Model file for the job. Use its own axes, mm. A direction names the side the tool comes from. Round coordinates to 2 decimals unless told otherwise and drop trailing zeros. Loops run counter-clockwise (first coordinate to the right, second up) from the corner with the lowest first, then second, coordinate; pieces in that order, holes last. Notation, with made-up numbers: M 78,54 L 114,54 A13 ccw 114,64 Z; hole C -15.5,50.25 d3. An arc over 180 degrees is marked long. Use a Markdown table: item, result. Add a question column.
Q1. Cut at D-D (x = 22). Give the cut face in (y, z).
Q2. Pin check, flat tips, straight feed: pin 1 (2 mm diameter, centred on x = 55, z = 23, fed in from -Y); pin 2 (20.5 mm diameter, centred on y = 32.5, z = 25, fed in from +X); pin 3 (1.5 mm diameter, centred on y = 52, z = 41, fed in from +X); pin 4 (8.5 mm diameter, centred on x = 49.6, z = 37.7, fed in from +Y). Stop position of each tip, or through.
Q3. Cut at A-A (z = 25). Give the cut face in (x, y) (3 decimals), plus the area to 3 significant figures.
Q4. Tool access for faces 4 (the face through (40, 2.997, 25)), 5 (the face through (41, 0, 25)): list every direction of +Z, -Z, +X, -X, +Y, -Y with a clear straight run to the whole face (end or side of a thin tool).
Q5. Probe line 1 (X direction, y = 42, z = 13.5); line 2 (Y direction, x = 1.65, z = 46.19). List the from-to ranges inside material, lowest first. Write a range as from..to.
Q6. Cut at B-B (y = 23.5). Give the cut face in (x, z), plus the area to 3 significant figures.
Q7. Cut at C-C (z = 30). Give the cut face in (x, y) (3 decimals), plus the area to 3 significant figures.
Q8. Mould opens along Y. For faces 1 (the face through (1, 59.995, 25)), 2 (the face through (21, 1, 50)), 3 (the face through (1.478, 21.233, 30.86)) say: +Y half, -Y half, draft (parallel to the pull), parting line (faces both ways), or undercut.
from build123d import *

# Parameters (mm, degrees)
BOSS_EXTRUDE1_DEPTH       = 50
SKETCH5_R                 = 3.2639
MOUNTING_HORIZONTAL_DEPTH = 107.647674169
SKETCH7_R                 = 12.7
BEARING_WITH_MOTOR_DEPTH  = 109.279157861
SKETCH8_R                 = 1.4732
F_4_40_WITH_MOTOR_DEPTH   = 109.279157861


with BuildPart() as part:
    # Sketch2 → Boss-Extrude1 (new body)
    with BuildSketch(Plane.XY):
        with BuildLine():
            Line((0, 5.842), (0, 59.9948))
            Line((0, 59.9948), (2.9972, 59.9948))
            Line((2.9972, 59.9948), (2.9972, 6.1722))
            ThreePointArc((2.9972, 6.1722), (3.92713597, 3.92713597), (6.1722, 2.9972))
            Line((6.1722, 2.9972), (75, 2.9972))
            Line((75, 2.9972), (75, 0))
            Line((75, 0), (5.842, 0))
            ThreePointArc((5.842, 0), (1.711082184, 1.711082184), (0, 5.842))
        make_face()
    extrude(amount=BOSS_EXTRUDE1_DEPTH)

    # Sketch5 → Mounting -- Horizontal (cut, through all)
    with BuildSketch(Plane(origin=(0, 2.9972, 0), x_dir=(1, 0, 0), z_dir=(0, 1, 0))):
        with Locations(Location((49.6, -12.3, 0), (0, 0, 270))):
            Circle(SKETCH5_R)
        with Locations(Location((49.6, -37.7, 0), (0, 0, 270))):
            Circle(SKETCH5_R)
    extrude(amount=-MOUNTING_HORIZONTAL_DEPTH, mode=Mode.SUBTRACT)

    # Sketch7 → Bearing -- With Motor (cut, through all)
    with BuildSketch(Plane.ZY):
        with Locations((25, 32.5)):
            Circle(SKETCH7_R)
    extrude(amount=-BEARING_WITH_MOTOR_DEPTH, mode=Mode.SUBTRACT)

    # Sketch8 → 4-40 -- With Motor (cut, through all)
    with BuildSketch(Plane.ZY):
        with Locations((3.81, 32.5)):
            Circle(SKETCH8_R)
        with Locations((46.19, 32.5)):
            Circle(SKETCH8_R)
    extrude(amount=-F_4_40_WITH_MOTOR_DEPTH, mode=Mode.SUBTRACT)


solid = part.part
Checked values:
| question | item | result |
|---|---|---|
| 1 | outline | M 0,0 L 3,0 L 3,50 L 0,50 Z |
| 2 | pin 1 | stops at y = 0 |
| 2 | pin 2 | passes through |
| 2 | pin 3 | stops at x = 3 |
| 2 | pin 4 | stops at y = 3 |
| 3 | outline | M 0,5.842 A5.842 ccw 5.842,0 L 75,0 L 75,2.997 L 6.172,2.997 A3.175 cw 2.997,6.172 L 2.997,19.8 L 0,19.8 Z; M 0,45.2 L 2.997,45.2 L 2.997,59.995 L 0,59.995 Z |
| 3 | area | 314 mm^2 |
| 4 | face 4 | +Z, -Z, +X, +Y |
| 4 | face 5 | +Z, -Z, +X, -X, -Y |
| 5 | line 1 | x = 0..3 |
| 5 | line 2 | y = 1.77..31.03, 33.97..59.99 |
| 6 | outline | M 0,0 L 3,0 L 3,16.04 L 0,16.04 Z; M 0,33.96 L 3,33.96 L 3,50 L 0,50 Z |
| 6 | area | 96.1 mm^2 |
| 7 | outline | M 0,5.842 A5.842 ccw 5.842,0 L 75,0 L 75,2.997 L 6.172,2.997 A3.175 cw 2.997,6.172 L 2.997,20.826 L 0,20.826 Z; M 0,44.174 L 2.997,44.174 L 2.997,59.995 L 0,59.995 Z |
| 7 | area | 320 mm^2 |
| 8 | face 1 | +Y half |
| 8 | face 2 | draft |
| 8 | face 3 | undercut |
